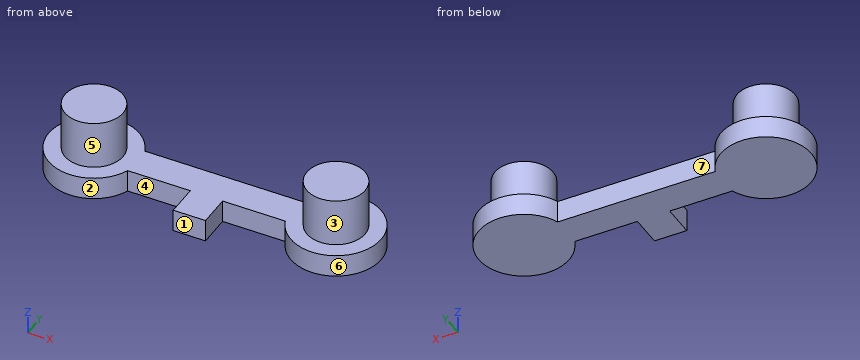
Autodesk Inventor part; units mm, degrees
ref_plane "YZ Plane" through (0, 0, 0) normal (1, 0, 0) x (0, 1, 0)
ref_plane "XZ Plane" through (0, 0, 0) normal (0, 1, 0) x (-1, 0, 0)
ref_plane "XY Plane" through (0, 0, 0) normal (0, 0, 1) x (1, 0, 0)
sketch "Эскиз1" plane through (0, 0, 0) normal (0, 0, 1) x (1, 0, 0)
  arc A0 (-4.8847, 1) -> (-4.8847, -1) centre (-7.5, 0) ccw
  arc A1 (4.8847, -1) -> (4.8847, 1) centre (7.5, 0) ccw
  line L0 (-7.5, 0) -> (7.5, 0) construction
  line L1 (-4.8847, 1) -> (4.8847, 1)
  line L2 (1, -1) -> (1, -3)
  line L3 (1, -3) -> (-1, -3)
  line L4 (-1, -3) -> (-1, -1)
  line L5 (-4.8847, -1) -> (-1, -1)
  line L6 (1, -1) -> (4.8847, -1)
  point P0 (0, 0)
  point P1 (0, 1)
  point P2 (0, -3)
  point P3 (0, 0)
  dimension "d0" = 5.6
  dimension "d1" = 5.6
  dimension "d2" = 15
  dimension "d3" = 1
  dimension "d7" = 2
  dimension "d8" = 2
extrude "Выдавливание1" add sketch "Эскиз1" along normal blind 1.4
sketch "Эскиз2" plane through (0, 0, 1.4) normal (0, 0, 1) x (1, 0, 0)
  arc A0 (-4.8847, 1) -> (-4.8847, -1) centre (-7.5, 0) ccw
  arc A1 (4.8847, -1) -> (4.8847, 1) centre (7.5, 0) ccw
  circle A2 centre (-7.5, 0) radius 1.8
  circle A3 centre (7.5, 0) radius 1.8
  point P0 (0, 0)
  dimension "d11" = 3.6
  dimension "d12" = 3.6
extrude "Выдавливание2" add sketch "Эскиз2" along normal blind 3
properties part number "fwd_rev_btns"
For this review, take the finished solid that the model builds, in its own axes (mm). Face numbers are marked on the shaded views. A direction names the side the tool comes from. Coordinates: 2 decimals unless noted, no trailing zeros. Loops run counter-clockwise (first coordinate to the right, second up) from the corner with the lowest first, then second, coordinate; pieces in that order, holes last. Notation, with made-up numbers: (53, -22) - (90, -22) arc R33 ccw to (90, 12) - close; hole circle Ø11 at (-38.75, 5). An arc over 180 degrees is marked (long way). Use one line per item in the form item = value. Start each with the question number.
1) Take a section at C-C (y = 0). State the section outline as (x, z) points, plus the area to 3 significant figures.
2) Draft analysis for pull direction X (two halves, no side actions). For the marked faces 1, 2 and 3, state which applies: released by +X, released by -X, zero draft, split by the parting line, or undercut.
3) For the marked faces 4, 5, 6 and 7, list the 3-axis set-ups (+Z, -Z, +X, -X, +Y, -Y) from which the entire face can be reached by the end or side of a thin tool; tool diameter is ignored.
4) Take a section at D-D (z = 2.2). State the section outline as (x, y) points, plus the area to 3 significant figures.
5) Take a section at A-A (x = -7.5). State the section outline as (y, z) points, plus the area to 3 significant figures.
6) For pin 1 (1.5 mm diameter, centred on x = -6.5, y = -1.5, fed in from -Z); pin 2 (0.7 mm diameter, centred on x = 0.5, z = 0.5, fed in from +Y); pin 3 (2 mm diameter, centred on y = 0.5, z = 4, fed in from -X); pin 4 (1.5 mm diameter, centred on y = 2, z = 4, fed in from +X), all flat-tipped, find the tip position at first contact; note any pin that passes through.
7) Take a section at B-B (z = 0.85). State the section outline as (x, y) points.
8) To check wall thickness, follow probe 1 along X at (y, z) = (-1.5, 0.95); probe 2 along Z at (x, y) = (-5.25, 0.05); probe 3 along X at (y, z) = (-2.1, 0.8). State the ranges of each line that lie inside material, in increasing order. Write a range as from..to.
From the geometry:
q1.outline = (-10.3, 0) - (10.3, 0) - (10.3, 1.4) - (9.3, 1.4) - (9.3, 4.4) - (5.7, 4.4) - (5.7, 1.4) - (-5.7, 1.4) - (-5.7, 4.4) - (-9.3, 4.4) - (-9.3, 1.4) - (-10.3, 1.4) - close
q1.area = 50.4 mm2
q2.face_1 = zero draft
q2.face_2 = undercut
q2.face_3 = undercut
q3.face_4 = +Z, -Z, -Y
q3.face_5 = +Z
q3.face_6 = +Z, -Z
q3.face_7 = +Z, -Z, +Y
q4.outline = circle Ø3.6 at (-7.5, 0); circle Ø3.6 at (7.5, 0)
q4.area = 20.4 mm2
q5.outline = (-2.8, 0) - (2.8, 0) - (2.8, 1.4) - (1.8, 1.4) - (1.8, 4.4) - (-1.8, 4.4) - (-1.8, 1.4) - (-2.8, 1.4) - close
q5.area = 18.6 mm2
q6.pin_1 = 0
q6.pin_2 = 1
q6.pin_3 = -9.3
q6.pin_4 = 8.8
q7.outline = (-4.88, -1) - (-1, -1) - (-1, -3) - (1, -3) - (1, -1) - (4.88, -1) arc R2.8 ccw (long way) to (4.88, 1) - (-4.88, 1) arc R2.8 ccw (long way) to start
q8.probe_1 = -9.86..-5.14, -1..1, 5.14..9.86
q8.probe_2 = 0..1.4
q8.probe_3 = -9.35..-5.65, -1..1, 5.65..9.35
